Geometry check sheet. Reference: the model listing, model coordinates, mm. A direction names the side the tool comes from. Round coordinates to 2 decimals unless told otherwise and drop trailing zeros. Loops run counter-clockwise (first coordinate to the right, second up) from the corner with the lowest first, then second, coordinate; pieces in that order, holes last. Notation, with made-up numbers: (11, 89.5) -> (55, 89.5) arc R24 ccw to (55, 125.5) -> close; hole circle Ø5 at (62, 59). An arc over 180 degrees is marked (long way). Use a Markdown table: item, result. Add a question column.
Q1. Sectioned sample at A-A, the plane y = -6. Enter the section's corners in (x, z), then the cut area to 3 significant figures.
Q2. Sectioned sample at D-D, the plane y = 15. Enter the section's corners in (x, z).
Q3. Release check for a two-part mould opening along Y. For faces 1 (the face through (0, -12, 13)), 2 (the face through (0, 7, -40)), 3 (the face through (-17.47, 14.81, -3.52)) record: released by +Y, released by -Y, zero draft, split by the parting line, or undercut.
Q4. Material ranges on L1, parallel to X at y = -1, z = -16.6; L2, parallel to Z at x = -21.25, y = 15; L3, parallel to X at y = 4.5, z = -16.6, recorded low to high.
Q5. Sectioned sample at C-C, the plane z = 0. Enter the section's corners in (x, y), then the cut area to 3 significant figures.
Q6. Sectioned sample at B-B, the plane x = 0. Enter the section's corners in (y, z).
Q7. Gauge pin test, flat ends, axial feed: P1, Ø9.5, axis at y = -8.5, z = -10.5, coming from the +X side; P2, Ø10, axis at x = -18, z = 29.5, coming from the -Y side; P3, Ø2, axis at y = 15, z = 0, coming from the -X side. Record the tip position at first contact, or that the pin passes through.
Q8. Set-up check for faces 4 (the face through (20, -5, -15)), 5 (the face through (-20, -5, 15)), 6 (the face through (0, 11.7, -4)), 7 (the face through (-22.101, 16.636, 0.215)): record each of +Z, -Z, +X, -X, +Y, -Y from which the full face is reachable in a straight line by a thin tool's end or side.
```python
from build123d import *

# Parameters (mm, degrees)
SKETCH1_W                   = 56
SKETCH1_H                   = 18
CHANNEL_BLOCK_DEPTH         = 40
SKETCH2_W                   = 40
SKETCH2_H                   = 12.5
CLAMP_UPPER_HALF_DEPTH      = 20
DOVETAIL_CHANNEL_DEPTH      = 34
DOVETAIL_CHANNEL_DEPTH_BACK = 41
HANDLEBAR_BORE_DEPTH        = 53.038447325
HANDLEBAR_BORE_DEPTH_BACK   = 53.038447325
SKETCH4_R                   = 12.1
M5_INSERT_HOLES_DEPTH       = 53.038447325
M5_INSERT_HOLES_DEPTH_BACK  = 53.038447325
SKETCH5_R                   = 3.2
SKETCH6_R                   = 1.65
LOCK_SCREW_HOLE_DEPTH       = 53.038447325


with BuildPart() as part:
    # Sketch1 → Channel Block (new, symmetric)
    with BuildSketch(Plane.XY):
        with Locations((0, 9)):
            Rectangle(SKETCH1_W, SKETCH1_H)
    extrude(amount=CHANNEL_BLOCK_DEPTH, both=True)

    # Sketch2 → Clamp Upper Half (add, symmetric)
    with BuildSketch(Plane(origin=(0, 0, 0), x_dir=(0, 0, -1), z_dir=(1, 0, 0))):
        with Locations((0, -5.75)):
            Rectangle(SKETCH2_W, SKETCH2_H)
    extrude(amount=CLAMP_UPPER_HALF_DEPTH, both=True)

    # Sketch3 → Dovetail Channel (cut, two sides: drawn at the far end of the back side and taken through both)
    with BuildSketch(Plane.XY.offset(-DOVETAIL_CHANNEL_DEPTH_BACK)):
        Polygon((-15.3, 18.5), (15.3, 18.5), (19.3, 11.7), (-19.3, 11.7), align=None)
    extrude(amount=DOVETAIL_CHANNEL_DEPTH + DOVETAIL_CHANNEL_DEPTH_BACK, mode=Mode.SUBTRACT)

    # Sketch4 → Handlebar Bore (cut, two sides: drawn at the far end of the back side and taken through both)
    with BuildSketch(Plane(origin=(0, 0, 0), x_dir=(0, 0, -1), z_dir=(1, 0, 0)).offset(-HANDLEBAR_BORE_DEPTH_BACK)):
        with Locations((0, -12)):
            Circle(SKETCH4_R)
    extrude(amount=HANDLEBAR_BORE_DEPTH + HANDLEBAR_BORE_DEPTH_BACK, mode=Mode.SUBTRACT)

    # Sketch5 → M5 Insert Holes (cut, two sides: drawn at the far end of the back side and taken through both)
    with BuildSketch(Plane(origin=(0, 0, 0), x_dir=(1, 0, 0), z_dir=(0, 1, 0)).offset(-M5_INSERT_HOLES_DEPTH_BACK)):
        with Locations(Location((0, -16.6, 0), (0, 0, 270))):
            Circle(SKETCH5_R)
        with Locations(Location((0, 16.6, 0), (0, 0, 270))):
            Circle(SKETCH5_R)
    extrude(amount=M5_INSERT_HOLES_DEPTH + M5_INSERT_HOLES_DEPTH_BACK, mode=Mode.SUBTRACT)

    # Sketch6 → Lock Screw Hole (cut, through all)
    with BuildSketch(Plane(origin=(0, 0, 0), x_dir=(0, 0, -1), z_dir=(1, 0, 0))):
        with Locations((0, 15)):
            Circle(SKETCH6_R)
    extrude(amount=-LOCK_SCREW_HOLE_DEPTH, mode=Mode.SUBTRACT)


solid = part.part
```
Values:
| question | item | result |
|---|---|---|
| 1 | outline | (-20, -20) -> (20, -20) -> (20, -10.51) -> (-20, -10.51) -> close; (-20, 10.51) -> (20, 10.51) -> (20, 20) -> (-20, 20) -> close; hole circle Ø6.4 at (0, -16.6); hole circle Ø6.4 at (0, 16.6) |
| 1 | area | 695 mm^2 |
| 2 | outline | (-28, -40) -> (-17.36, -40) -> (-17.36, -1.65) -> (-28, -1.65) -> close; (-28, 1.65) -> (-17.36, 1.65) -> (-17.36, 34) -> (17.36, 34) -> (17.36, -40) -> (28, -40) -> (28, 40) -> (-28, 40) -> close |
| 3 | face 1 | released by -Y |
| 3 | face 2 | zero draft |
| 3 | face 3 | undercut |
| 4 | L1 | -20 to -3.2, 3.2 to 20 |
| 4 | L2 | -40 to -1.65, 1.65 to 40 |
| 4 | L3 | -28 to -3.2, 3.2 to 28 |
| 5 | outline | (-28, 0.1) -> (28, 0.1) -> (28, 18) -> (15.59, 18) -> (19.3, 11.7) -> (-19.3, 11.7) -> (-18.33, 13.35) -> (-28, 13.35) -> close; (-28, 16.65) -> (-16.39, 16.65) -> (-15.59, 18) -> (-28, 18) -> close |
| 5 | area | 747 mm^2 |
| 6 | outline | (-12, -20) -> (0, -20) -> (0, -40) -> (11.7, -40) -> (11.7, -19.8) -> (-12, -19.8) -> close; (-12, -13.4) -> (11.7, -13.4) -> (11.7, 13.4) -> (-12, 13.4) -> (-12, 12.1) arc R12.1 cw to (-12, -12.1) -> close; (-12, 19.8) -> (11.7, 19.8) -> (11.7, 34) -> (18, 34) -> (18, 40) -> (0, 40) -> (0, 20) -> (-12, 20) -> close |
| 7 | P1 | x = 20 |
| 7 | P2 | y = 0 |
| 7 | P3 | x = 16.77 |
| 8 | face 4 | +Z, -Z, +X, -Y |
| 8 | face 5 | +Z, -Z, -X, -Y |
| 8 | face 6 | -Z |
| 8 | face 7 | -X |
